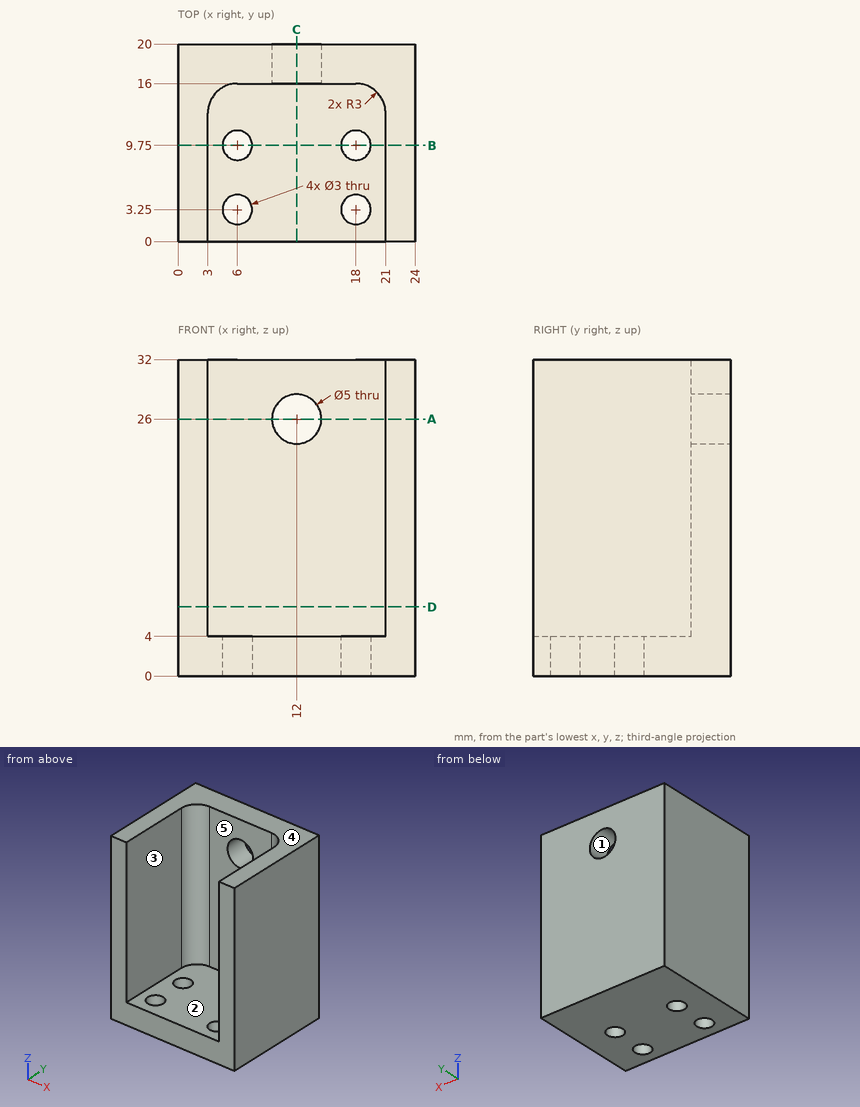
Job drawing, mm, ordinate dimensions from the low corner. One solid piece. A direction names the side the tool comes from. Coordinates: 2 decimals unless noted, no trailing zeros. Order: outer loops, then holes, each group sorted by start corner. A loop starts at its lowest first (then second) coordinate and runs counter-clockwise, first axis right, second up. Notation, with made-up numbers: (42.5, 65) - (86.5, 65) arc R30 ccw to (86.5, 94) - close; hole circle Ø1 at (23, 5). An arc over 180 degrees is marked (long way). Return JSON: item names as keys, results as strings. Group by question number.
1) Saw through at C-C, the plane x = 12. Write the cut outline in (y, z).
2) Saw through at A-A, the plane z = 26. Write the cut outline in (x, y), plus the area to 3 significant figures.
3) Tool access for the marked faces 4 and 5: list every direction of +Z, -Z, +X, -X, +Y, -Y with a clear straight run to the whole face (end or side of a thin tool).
4) Mould opens along Z. For the marked faces 1, 2 and 3 say: released by +Z, released by -Z, zero draft, split by the parting line, or undercut.
5) Saw through at B-B, the plane y = 9.75. Write the cut outline in (x, z).
6) Saw through at D-D, the plane z = 7. Write the cut outline in (x, y), plus the area to 3 significant figures.
7) Flat gauge pins, fed straight in: P1, Ø2.5, axis at x = 6, y = 3.25, coming from the +Z side; P2, Ø2, axis at x = 4.5, z = 19.5, coming from the -Y side; P3, Ø8, axis at x = 19.5, z = 6.5, coming from the -Y side; P4, Ø6, axis at x = 15.5, y = 8, coming from the +Z side. Where does each tip first touch, or does it go through?
8) Probe line 1 (Y direction, x = 18, z = 2.05); line 2 (X direction, y = 13, z = 29); line 3 (Y direction, x = 14.5, z = 30). List the from-to ranges inside material, lowest first. Write a range as from..to.
Values found:
{
 "1": {"outline": "(0, 0) - (20, 0) - (20, 23.5) - (16, 23.5) - (16, 4) - (0, 4) - close; (16, 28.5) - (20, 28.5) - (20, 32) - (16, 32) - close"},
 "2": {"outline": "(0, 0) - (3, 0) - (3, 13) arc R3 cw to (6, 16) - (9.5, 16) - (9.5, 20) - (0, 20) - close; (14.5, 16) - (18, 16) arc R3 cw to (21, 13) - (21, 0) - (24, 0) - (24, 20) - (14.5, 20) - close", "area": "176 mm²"},
 "3": {"face 4": "+Z, +X, -X, +Y, -Y", "face 5": "+Z, -Y"},
 "4": {"face 1": "undercut", "face 2": "released by +Z", "face 3": "zero draft"},
 "5": {"outline": "(0, 0) - (4.5, 0) - (4.5, 4) - (3, 4) - (3, 32) - (0, 32) - close; (7.5, 0) - (16.5, 0) - (16.5, 4) - (7.5, 4) - close; (19.5, 0) - (24, 0) - (24, 32) - (21, 32) - (21, 4) - (19.5, 4) - close"},
 "6": {"outline": "(0, 0) - (3, 0) - (3, 13) arc R3 cw to (6, 16) - (18, 16) arc R3 cw to (21, 13) - (21, 0) - (24, 0) - (24, 20) - (0, 20) - close", "area": "196 mm²"},
 "7": {"P1": "passes through", "P2": "stops at y = 14.66", "P3": "stops at y = 0", "P4": "stops at z = 4"},
 "8": {"line 1": "y = 0..1.75, 4.75..8.25, 11.25..20", "line 2": "x = 0..3, 21..24", "line 3": "y = 16..20"}
}
